from build123d import *

# Parameters (mm, degrees)
F0_W     = 25.4
F0_H     = 25.4
F1_DEPTH = 9.525
F2_W     = 3
F2_H     = 15
F3_DEPTH = 18
F4_R     = 7.49999
F5_W     = 12.7
F5_H     = 3.175
F6_DEPTH = 25.401
F7_W     = 12.7
F7_H     = 3.175
F8_DEPTH = 25.401
F10_D    = 5
F11_R    = 5.08
F12_R    = 0.254


# Not quite as in the source:
# - a fillet or chamfer is up to 0.001 mm smaller than in the source, because OpenCascade refuses the exact size


with BuildPart() as f1:
    # F0 (on Top) → F1 (new body)
    with BuildSketch(Plane.XY):
        Rectangle(F0_W, F0_H)
    extrude(amount=F1_DEPTH)

    # F2 (on face) → F3 (join)
    with BuildSketch(Plane.XY.offset(9.525)):
        with Locations((-3.2, 0)):
            Rectangle(F2_W, F2_H)
        with Locations((3.2, 0)):
            Rectangle(F2_W, F2_H)
    extrude(amount=F3_DEPTH)

    # F4 (radius 7.5 in the source; OpenCascade refuses exactly that, so slightly less here)
    f4_edges = [f1.edges().sort_by_distance(p)[0] for p in [
        (3.2, 7.5, 27.525),
        (3.2, -7.5, 27.525),
        (-3.2, 7.5, 27.525),
        (-3.2, -7.5, 27.525),
    ]]
    fillet(f4_edges, radius=F4_R)

    # F5 (on face) → F6 (cut, through all)
    with BuildSketch(Plane.YZ.offset(12.7)):
        with Locations((0, 3.175)):
            Rectangle(F5_W, F5_H)
    extrude(amount=-F6_DEPTH, mode=Mode.SUBTRACT)

    # F7 (on face) → F8 (cut, through all)
    with BuildSketch(Plane.XZ.offset(12.7)):
        with Locations((0, 6.35)):
            Rectangle(F7_W, F7_H)
    extrude(amount=-F8_DEPTH, mode=Mode.SUBTRACT)

    # F10 (through all)
    with Locations(Plane.YZ.offset(4.7)):
        with Locations((0, 20.025)):
            Hole(F10_D / 2)

    # F11
    f11_edges = [f1.edges().sort_by_distance(p)[0] for p in [
        (12.7, -12.7, 4.7625),
        (-12.7, -12.7, 4.7625),
        (12.7, 12.7, 4.7625),
        (-12.7, 12.7, 4.7625),
    ]]
    fillet(f11_edges, radius=F11_R)

    # F12
    f12_edges = [f1.edges().sort_by_distance(p)[0] for p in [
        (0, -12.7, 4.7625),
        (12.7, 0, 1.5875),
        (0, 12.7, 4.7625),
        (-12.7, 0, 1.5875),
    ]]
    fillet(f12_edges, radius=F12_R)


solid = f1.part
Can you work these out from the model? Positions are in its coordinate system, mm. A direction names the side the tool comes from. Give positions to 0.01 mm unless a question says otherwise; leave off trailing zeros. Order: outer loops, then holes, each group sorted by start corner. A loop starts at its lowest first (then second) coordinate and runs counter-clockwise, first axis right, second up. Notation, with made-up numbers: M 35,45 L 72,45 A29 ccw 72,73 Z; hole C -10,83.25 d11. An arc over 180 degrees is marked long. One line per item, written item: value.
Item 1: For faces 4 (the face through (3, 7.5, 15)), 5 (the face through (3, -7.5, 15)), 6 (the face through (1.7, 0, 16)), which set-ups out of +Z, -Z, +X, -X, +Y, -Y let a thin tool reach every point of the face, with its end or its side?
Verdict:
face 4: +Z, +X, -X, +Y
face 5: +Z, +X, -X, -Y
face 6: +Z, +Y, -Y
Item 2: If we section it at B-B on x = -3.25: State how many separate pieces and enclosed holes the cut face has, and give its area (3 significant figures).
Verdict:
separate pieces: 2
enclosed holes: 1
area: 347 mm2
Item 3: If we section it at A-A on z = 11.75: Write out the boundary of the cut face in (x, y).
Verdict:
outline: M -4.7,-7.5 L -1.7,-7.5 L -1.7,7.5 L -4.7,7.5 Z; M 1.7,-7.5 L 4.7,-7.5 L 4.7,7.5 L 1.7,7.5 Z
Item 4: If we mould it in two halves opening along Y, with no side actions, what happens to faces 1 (the face through (0, 0, 1.588)), 2 (the face through (3.22, -5.36, 25.27)), 3 (the face through (0, 12.7, 4))? For each: pulls with the +Y half, pulls with the -Y half, needs draft (parallel to the pull), parting line crosses it, or undercut.
Verdict:
face 1: undercut
face 2: pulls with the -Y half
face 3: pulls with the +Y half
Item 5: Please list where these lines run through material, in increasing order: line 1 (X direction, y = 0.25, z = 23.25); line 2 (Z direction, x = -4.25, y = 9.5) (1 decimal); line 3 (Z direction, x = 3.6, y = 0) (1 decimal).
Verdict:
line 1: -4.7 to -1.7, 1.7 to 4.7
line 2: 0 to 4.8, 7.9 to 9.5
line 3: 0 to 1.6, 7.9 to 17.5, 22.5 to 27.5
Item 6: For pin 1 (4 mm diameter, centred on x = -9, z = 7.5, fed in from +Y); pin 2 (8 mm diameter, centred on y = -2, z = 22, fed in from -X); pin 3 (3.5 mm diameter, centred on x = -3, z = 14.5, fed in from -Y); pin 4 (2 mm diameter, centred on y = -9.5, z = 9, fed in from +X), each with a flat end and sliding along its axis, tell me the tip position at first contact or that it passes through.
Verdict:
pin 1: y = 12.7
pin 2: x = -4.7
pin 3: y = -7.5
pin 4: x = 12.62
Item 7: If we section it at D-D on z = 19: Write out the boundary of the cut face in (x, y).
Verdict:
outline: M -4.7,-7.5 L -1.7,-7.5 L -1.7,-2.28 L -4.7,-2.28 Z; M -4.7,2.28 L -1.7,2.28 L -1.7,7.5 L -4.7,7.5 Z; M 1.7,-7.5 L 4.7,-7.5 L 4.7,-2.28 L 1.7,-2.28 Z; M 1.7,2.28 L 4.7,2.28 L 4.7,7.5 L 1.7,7.5 Z
